Design review of the part shown in the three views and the two pictorial views. Dimensions are in mm from the part's minimum x, y and z. A direction names the side the tool comes from. Round coordinates to 2 decimals unless told otherwise and drop trailing zeros. Write each loop counter-clockwise with the first axis right and the second up, starting at its lowest first coordinate (ties: lowest second). Pieces come first, ordered by that corner, then holes. Notation, with made-up numbers: (48.5, -36) - (67.5, -36) arc R13 ccw to (67.5, -26) - close; hole circle Ø3 at (57, -25). An arc over 180 degrees is marked (long way). Use one line per item in the form item = value.
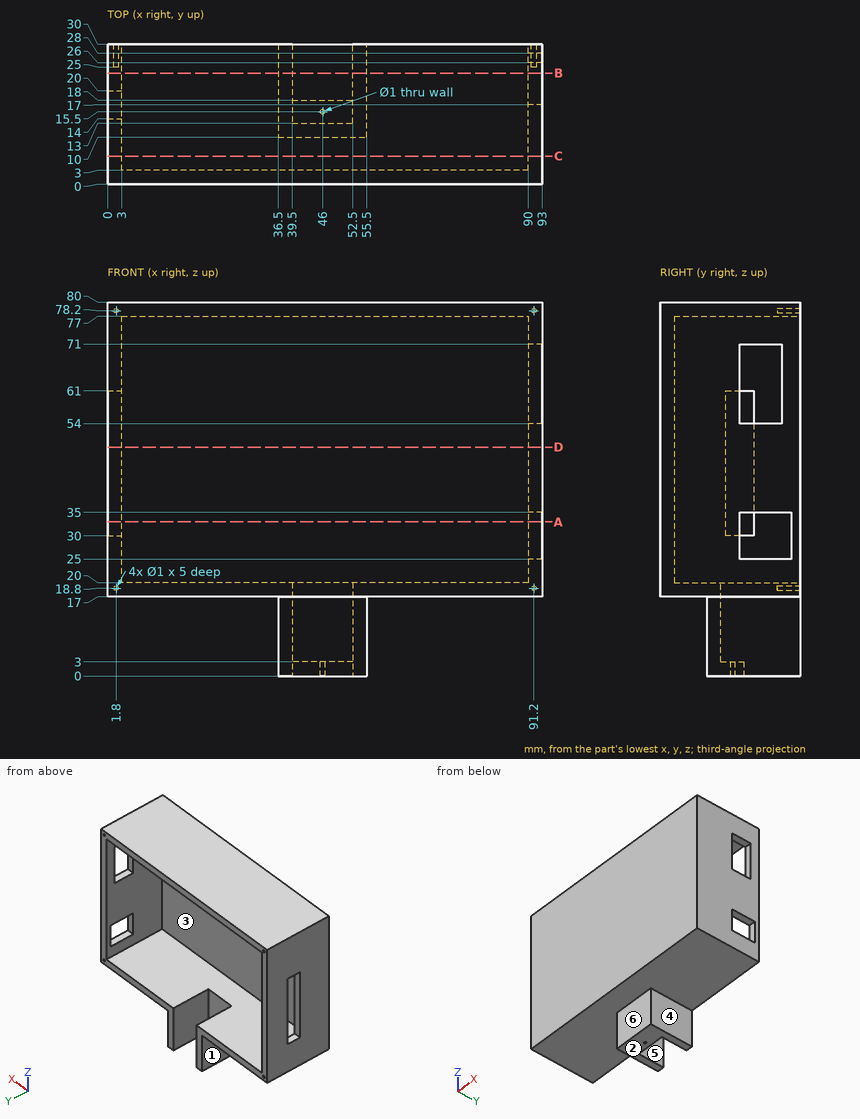
Q1. We need section D-D on z = 49. Write out the cut boundary in (x, y), then the cut area to 3 significant figures.
Calculated:
outline = (0, 0) - (93, 0) - (93, 30) - (90, 30) - (90, 3) - (3, 3) - (3, 14) - (0, 14) - close; (0, 20) - (3, 20) - (3, 30) - (0, 30) - close
area = 423 mm2
Q2. For P1, Ø0.9, axis at x = 44.5, z = 2, coming from the +Y side; P2, Ø9, axis at x = 31.5, y = 13, coming from the -Z side; P3, Ø8, axis at x = 67, z = 50, coming from the +Y side, all flat-tipped, find the tip position at first contact; note any pin that passes through.
Calculated:
P1 = 18
P2 = 17
P3 = 3
Q3. We need section A-A on z = 33. Write out the cut boundary in (x, y), then the cut area to 3 significant figures.
Calculated:
outline = (0, 0) - (93, 0) - (93, 17) - (90, 17) - (90, 3) - (3, 3) - (3, 14) - (0, 14) - close; (0, 20) - (3, 20) - (3, 30) - (0, 30) - close; (90, 28) - (93, 28) - (93, 30) - (90, 30) - close
area = 390 mm2
Q4. Machinability: for the marked faces 4, 5 and 6, which of the approach directions +Z, -Z, +X, -X, +Y, -Y give a long, thin tool a straight path to every point of the face, cutting with its end or side? Answer none if there is none.
Calculated:
face_4 = -Z, +X, +Y, -Y
face_5 = +Y
face_6 = -Z, +X, -X, -Y
Q5. To check wall thickness, follow line 1 along Z through (x, y) = (91.2, 28.85); line 2 along Z through (x, y) = (91.2, 27.6); line 3 along X through (y, z) = (27.8, 78.2). State the ranges of each line that lie inside material, in increasing order. Write a range as from..to.
Calculated:
line_1 = 17..18.3, 19.3..77.7, 78.7..80
line_2 = 17..18.3, 19.3..25, 35..77.7, 78.7..80
line_3 = 0..1.3, 2.3..90.7, 91.7..93
Q6. We need section B-B on y = 23.75. Write out the cut boundary in (x, z).
Calculated:
outline = (0, 17) - (36.5, 17) - (36.5, 0) - (39.5, 0) - (39.5, 20) - (3, 20) - (3, 77) - (90, 77) - (90, 71) - (93, 71) - (93, 80) - (0, 80) - close; (52.5, 0) - (55.5, 0) - (55.5, 17) - (93, 17) - (93, 25) - (90, 25) - (90, 20) - (52.5, 20) - close; (90, 35) - (93, 35) - (93, 54) - (90, 54) - close
Q7. Draft analysis for pull direction Z (two halves, no side actions). For the marked faces 1, 2 and 3, state which applies: released by +Z, released by -Z, zero draft, split by the parting line, or undercut.
Calculated:
face_1 = zero draft
face_2 = released by -Z
face_3 = undercut
Q8. We need section C-C on y = 6. Write out the cut boundary in (x, z).
Calculated:
outline = (0, 17) - (93, 17) - (93, 80) - (0, 80) - close; hole (3, 20) - (90, 20) - (90, 77) - (3, 77) - close
